The drawing under review shows one solid part. Ordinate dimensions are in mm from its lowest x, y, z. A direction names the side the tool comes from. Coordinates: 2 decimals unless noted, no trailing zeros. Order: outer loops, then holes, each group sorted by start corner. A loop starts at its lowest first (then second) coordinate and runs counter-clockwise, first axis right, second up. Notation, with made-up numbers: (61.25, 57) - (114.25, 57) arc R19 cw to (114.25, 63) - close; hole circle Ø2 at (24, -4.5). An arc over 180 degrees is marked (long way). Answer in a Markdown table with one row per item.
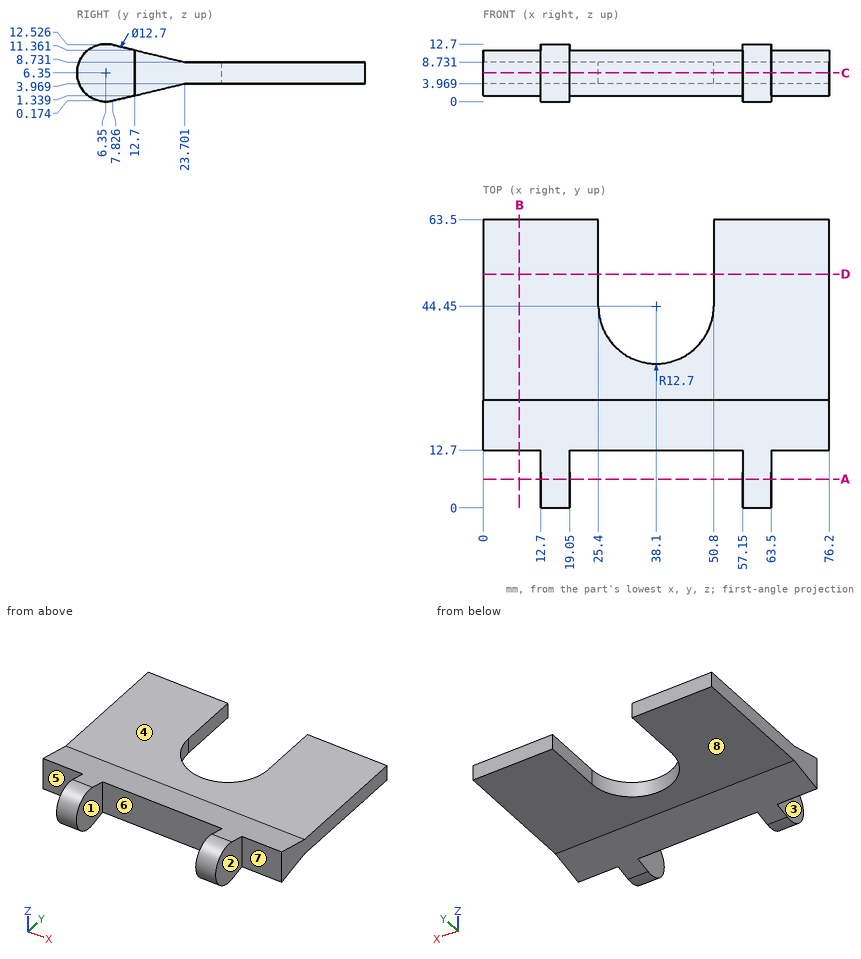
Item 1: We need section C-C, the plane z = 6.35. Write out the cut boundary in (x, y).
Check values:
| item | result |
|---|---|
| outline | (0, 12.7) - (12.7, 12.7) - (12.7, 0) - (19.05, 0) - (19.05, 12.7) - (57.15, 12.7) - (57.15, 0) - (63.5, 0) - (63.5, 12.7) - (76.2, 12.7) - (76.2, 63.5) - (50.8, 63.5) - (50.8, 44.45) arc R12.7 cw to (25.4, 44.45) - (25.4, 63.5) - (0, 63.5) - close |
Item 2: Tool access review of the marked faces 4, 5, 6, 7 and 8: name each direction out of +Z, -Z, +X, -X, +Y, -Y from which nothing blocks a thin tool from reaching the whole face with its end or side.
Check values:
| item | result |
|---|---|
| face 4 | +Z, +X, -X, +Y |
| face 5 | +Z, -Z, -X, -Y |
| face 6 | +Z, -Z, -Y |
| face 7 | +Z, -Z, +X, -Y |
| face 8 | -Z, +X, -X, +Y |
Item 3: We need section B-B, the plane x = 8. Write out the cut boundary in (y, z), then the cut area to 3 significant figures.
Check values:
| item | result |
|---|---|
| outline | (12.7, 1.34) - (23.7, 3.97) - (63.5, 3.97) - (63.5, 8.73) - (23.7, 8.73) - (12.7, 11.36) - close |
| area | 271 mm^2 |
Item 4: We need section A-A, the plane y = 6.35. Write out the cut boundary in (x, z).
Check values:
| item | result |
|---|---|
| outline | (12.7, 0) - (19.05, 0) - (19.05, 12.7) - (12.7, 12.7) - close; (57.15, 0) - (63.5, 0) - (63.5, 12.7) - (57.15, 12.7) - close |
Item 5: Mouldability with a two-part tool opening along X and no side actions: class the marked faces 1, 2 and 3 as +X half, -X half, draft (parallel to the pull), parting line (faces both ways), or undercut.
Check values:
| item | result |
|---|---|
| face 1 | undercut |
| face 2 | +X half |
| face 3 | -X half |
Item 6: To check wall thickness, follow line 1 (X direction, y = 58, z = 4.5); line 2 (X direction, y = 5, z = 3); line 3 (Y direction, x = 19.5, z = 4). State the ranges of each line that lie inside material, in increasing order. Write a range as from..to.
Check values:
| item | result |
|---|---|
| line 1 | 0..25.4, 50.8..76.2 |
| line 2 | 12.7..19.05, 57.15..63.5 |
| line 3 | 12.7..63.5 |
Item 7: We need section D-D, the plane y = 51.5. Write out the cut boundary in (x, z), then the cut area to 3 significant figures.
Check values:
| item | result |
|---|---|
| outline | (0, 3.97) - (25.4, 3.97) - (25.4, 8.73) - (0, 8.73) - close; (50.8, 3.97) - (76.2, 3.97) - (76.2, 8.73) - (50.8, 8.73) - close |
| area | 242 mm^2 |
Item 8: Clearance check with flat-ended pins moving along their axes: pin 1 Ø3 at (x, z) = (8.5, 4.5) entering from -Y; pin 2 Ø20 at (x, y) = (22, 43.5) entering from +Z; pin 3 Ø4 at (x, y) = (28, 28.5) entering from -Z. State where each tip first meets the part, or that it passes through.
Check values:
| item | result |
|---|---|
| pin 1 | y = 12.7 |
| pin 2 | z = 8.73 |
| pin 3 | z = 3.97 |
